```python
from build123d import *

# Parameters (mm, degrees)
SKETCH1_W                = 141
SKETCH1_H                = 15
BOSS_EXTRUDE1_DEPTH      = 1.5
SKETCH2_W                = 30
SKETCH2_H                = 3
SKETCH2_W_2              = 17
BOSS_EXTRUDE2_DEPTH      = 1.5
SKETCH12_W               = 25
SKETCH12_H               = 3
BOSS_EXTRUDE3_DEPTH      = 1.5
SKETCH13_W               = 35
SKETCH13_H               = 3
BOSS_EXTRUDE4_DEPTH      = 1.5
SKETCH15_W               = 11
SKETCH15_H               = 9
CUT_EXTRUDE10_DEPTH      = 2.5
CUT_EXTRUDE10_DEPTH_BACK = 2.5
FILLET4_R                = 2
CUT_EXTRUDE11_DEPTH      = 2.5
CUT_EXTRUDE11_DEPTH_BACK = 2.5
SKETCH17_W               = 3
SKETCH17_H               = 6
CUT_EXTRUDE12_DEPTH      = 2.5
CUT_EXTRUDE12_DEPTH_BACK = 2.5


with BuildPart() as part:
    # Sketch1 → Boss-Extrude1 (new body, symmetric)
    with BuildSketch(Plane(origin=(0, 0, 0), x_dir=(1, 0, 0), z_dir=(0, 1, 0))):
        Rectangle(SKETCH1_W, SKETCH1_H)
    extrude(amount=BOSS_EXTRUDE1_DEPTH, both=True)

    # Sketch2 → Boss-Extrude2 (add, symmetric)
    with BuildSketch(Plane(origin=(0, 0, 0), x_dir=(1, 0, 0), z_dir=(0, 1, 0))):
        with Locations((25.5, -9)):
            Rectangle(SKETCH2_W, SKETCH2_H)
        with Locations((62, -9)):
            Rectangle(SKETCH2_W_2, SKETCH2_H)
    extrude(amount=BOSS_EXTRUDE2_DEPTH, both=True)

    # Sketch12 → Boss-Extrude3 (add, symmetric)
    with BuildSketch(Plane(origin=(0, 0, 0), x_dir=(1, 0, 0), z_dir=(0, 1, 0))):
        with Locations((-38, -9)):
            Rectangle(SKETCH12_W, SKETCH12_H)
    extrude(amount=BOSS_EXTRUDE3_DEPTH, both=True)

    # Sketch13 → Boss-Extrude4 (add, symmetric)
    with BuildSketch(Plane(origin=(0, 0, 0), x_dir=(1, 0, 0), z_dir=(0, 1, 0))):
        with Locations((-28, 9)):
            Rectangle(SKETCH13_W, SKETCH13_H)
        with Locations((28, 9)):
            Rectangle(SKETCH13_W, SKETCH13_H)
    extrude(amount=BOSS_EXTRUDE4_DEPTH, both=True)

    # Sketch15 → Cut-Extrude10 (cut, two sides)
    with BuildSketch(Plane(origin=(0, 0, 0), x_dir=(1, 0, 0), z_dir=(0, 1, 0))) as cut_extrude10_sk:
        with Locations((62, 0)):
            Rectangle(SKETCH15_W, SKETCH15_H)
    extrude(amount=CUT_EXTRUDE10_DEPTH, mode=Mode.SUBTRACT)
    extrude(cut_extrude10_sk.sketch, amount=-CUT_EXTRUDE10_DEPTH_BACK, mode=Mode.SUBTRACT)

    # Fillet4
    fillet4_edges = [part.edges().sort_by_distance(p)[0] for p in [
        (56.5, 0, 4.5),
        (56.5, 0, -4.5),
        (67.5, 0, -4.5),
        (67.5, 0, 4.5),
    ]]
    fillet(fillet4_edges, radius=FILLET4_R)

    # Sketch16 → Cut-Extrude11 (cut, two sides)
    with BuildSketch(Plane(origin=(0, 0, 0), x_dir=(1, 0, 0), z_dir=(0, 1, 0))) as cut_extrude11_sk:
        Polygon((49, 3.299038106), (47.700961894, 1.049038106), (50.299038106, 1.049038106), align=None)
        Polygon((50.5, -1.799038106), (48.25, -0.5), (48.25, -3.098076211), align=None)
    extrude(amount=CUT_EXTRUDE11_DEPTH, mode=Mode.SUBTRACT)
    extrude(cut_extrude11_sk.sketch, amount=-CUT_EXTRUDE11_DEPTH_BACK, mode=Mode.SUBTRACT)

    # Sketch17 → Cut-Extrude12 (cut, two sides)
    with BuildSketch(Plane(origin=(0, 0, 0), x_dir=(1, 0, 0), z_dir=(0, 1, 0))) as cut_extrude12_sk:
        with Locations((-69, 0)):
            Rectangle(SKETCH17_W, SKETCH17_H)
    extrude(amount=CUT_EXTRUDE12_DEPTH, mode=Mode.SUBTRACT)
    extrude(cut_extrude12_sk.sketch, amount=-CUT_EXTRUDE12_DEPTH_BACK, mode=Mode.SUBTRACT)


solid = part.part
```
Geometry: final body of the model. Coordinates: model frame, mm. A direction names the side the tool comes from. Give positions to 0.01 mm unless a question says otherwise; leave off trailing zeros. Loops run counter-clockwise (first coordinate to the right, second up) from the corner with the lowest first, then second, coordinate; pieces in that order, holes last. Notation, with made-up numbers: (85, 75) - (122, 75) arc R26 cw to (122, 101) - close; hole circle Ø1 at (51.25, 54). An arc over 180 degrees is marked (long way). Answer as CSV lines item,"result". Start each with the question number.
(1) Pin query (flat end, axial travel): P1, Ø0.9, axis at y = 0, z = 1.5, coming from the -X side; P2, Ø0.9, axis at y = 0.5, z = -9.5, coming from the -X side; P3, Ø0.9, axis at x = -64, y = -0.5, coming from the -Z side. Return the tip coordinate at first contact, or that it passes through.
(2) Section query C-C (x = -19). Output: boundary loops of the cut face in (y, z).
(3) Section query A-A (x = -2). Output: boundary loops of the cut face in (y, z), and give its area (3 significant figures).
(4) Reachability of faces 5 (the face through (56.5, 0, 0)), 6 (the face through (10.5, 0, -9)), 7 (the face through (40.5, 0, 9)) from +Z, -Z, +X, -X, +Y, -Y: full face, straight path, thin tool, end or side. Return the list, or none.
(5) Ray query, line 1 along X through (y, z) = (0.5, 7.75); line 2 along X through (y, z) = (-0.05, -1.75); line 3 along X through (y, z) = (1.05, -4). Return the intervals inside material, ascending. Write a range as [from, to].
(6) Mould query, pull axis X, two halves, no side actions, for faces 1 (the face through (-58, 0, -7.5)), 2 (the face through (0, 0, -7.5)), 3 (the face through (48.25, 0, 2)), 4 (the face through (-67.5, 0, 0)). Classes: +X half, -X half, draft (parallel to the pull), parting line (faces both ways), or undercut.
(7) Section query B-B (y = -0.7). Give the number of separate pieces and of enclosed holes in the cut face, and give its area (3 significant figures).
Worked answers:
1,P1,"stops at x = -67.5"
1,P2,"stops at x = -45.5"
1,P3,"stops at z = -7.5"
2,outline,"(-1.5, -10.5) - (1.5, -10.5) - (1.5, 7.5) - (-1.5, 7.5) - close"
3,outline,"(-1.5, -7.5) - (1.5, -7.5) - (1.5, 7.5) - (-1.5, 7.5) - close"
3,area,"45.0 mm^2"
4,face 5,"+Y, -Y"
4,face 6,"-Z, +Y, -Y"
4,face 7,"+Z, +Y, -Y"
5,line 1,"x = [-50.5, -25.5], [10.5, 40.5], [53.5, 70.5]"
5,line 2,"x = [-67.5, 48.11], [49.89, 56.5], [67.5, 70.5]"
5,line 3,"x = [-70.5, 57.18], [66.82, 70.5]"
6,face 1,"draft"
6,face 2,"undercut"
6,face 3,"undercut"
6,face 4,"-X half"
7,separate pieces,"1"
7,enclosed holes,"3"
7,area,"2,420 mm^2"
